Build history of the part. All positions in model axes, mm. Round coordinates to 2 decimals unless told otherwise and drop trailing zeros. Loops run counter-clockwise (first coordinate to the right, second up) from the corner with the lowest first, then second, coordinate; pieces in that order, holes last. Notation, with made-up numbers: (56, 35.5) - (95, 35.5) arc R13 cw to (95, 44.5) - close; hole circle Ø4 at (43, 43.5). An arc over 180 degrees is marked (long way). Use a Markdown table: item, result.
from build123d import *

# Parameters (mm, degrees)
F0_R     = 12.5
F1_DEPTH = 600
F2_SIZE  = 1
F3_SIZE  = 1


with BuildPart() as f1:
    # F0 (on Front) → F1 (new body)
    with BuildSketch(Plane.XZ):
        Circle(F0_R)
    extrude(amount=F1_DEPTH)

    # F2
    f2_edges = [f1.edges().sort_by_distance(p)[0] for p in [
        (-12.5, -600, 0),
    ]]
    chamfer(f2_edges, length=F2_SIZE)

    # F3
    f3_edges = [f1.edges().sort_by_distance(p)[0] for p in [
        (-12.5, 0, 0),
    ]]
    chamfer(f3_edges, length=F3_SIZE)


solid = f1.part
Q1. Drop flat-ended pins along their axis: pin 1 (1.5 mm diameter, centred on x = 7.5, y = -400.5, fed in from +Z); pin 2 (6 mm diameter, centred on y = -402, z = 9.5, fed in from +X); pin 3 (1.5 mm diameter, centred on x = -3.5, y = -67.5, fed in from +Z). Give the stop position or say it passes through.
Results found:
| item | result |
|---|---|
| pin 1 | stops at z = 10.52 |
| pin 2 | stops at x = 10.68 |
| pin 3 | stops at z = 12.19 |
Q2. Cut at A-A, the plane y = -534. List the corners of the cut face in (x, z).
Results found:
| item | result |
|---|---|
| outline | circle Ø25 at (0, 0) |
Q3. Probe line 1 (Z direction, x = 1, y = -401); line 2 (X direction, y = -224.5, z = 1.5). List the from-to ranges inside material, lowest first.
Results found:
| item | result |
|---|---|
| line 1 | z = -12.46 to 12.46 |
| line 2 | x = -12.41 to 12.41 |
